Design review of the part built by this model. Coordinates are the model's own, in mm. A direction names the side the tool comes from. Coordinates: 2 decimals unless noted, no trailing zeros. Loops run counter-clockwise (first coordinate to the right, second up) from the corner with the lowest first, then second, coordinate; pieces in that order, holes last. Notation, with made-up numbers: (81, 71) -> (101, 71) arc R15 cw to (101, 91) -> close; hole circle Ø7 at (15, -8.75). An arc over 180 degrees is marked (long way). Use CSV: the item, a comma, the result in double quotes.
```python
from build123d import *

# Parameters (mm, degrees)
SKETCH2_W                                           = 240
SKETCH2_H                                           = 140
EXTRUDE1_DEPTH                                      = 12
CBORE_FOR_M4_HEX_SOCKET_HEAD_CAP_SCREW1_D           = 4.5
CBORE_FOR_M4_HEX_SOCKET_HEAD_CAP_SCREW1_CBORE_D     = 8
CBORE_FOR_M4_HEX_SOCKET_HEAD_CAP_SCREW1_CBORE_DEPTH = 4.4
CBORE_FOR_M6_HEX_SOCKET_HEAD_CAP_SCREW1_D           = 6.6
CBORE_FOR_M6_HEX_SOCKET_HEAD_CAP_SCREW1_CBORE_D     = 11
CBORE_FOR_M6_HEX_SOCKET_HEAD_CAP_SCREW1_CBORE_DEPTH = 6.4
CBORE_FOR_M6_HEX_SOCKET_HEAD_CAP_SCR_2_COUNT        = 2
CBORE_FOR_M6_HEX_SOCKET_HEAD_CAP_SCR_2_PITCH        = 35


with BuildPart() as part:
    # Sketch2 → Extrude1 (new body)
    with BuildSketch(Plane(origin=(0, 0, 0), x_dir=(1, 0, 0), z_dir=(0, 1, 0))):
        Rectangle(SKETCH2_W, SKETCH2_H)
    extrude(amount=EXTRUDE1_DEPTH)

    # CBORE for M4 Hex Socket Head Cap Screw1 (through all)
    with Locations(Plane(origin=(0, 12, 0), x_dir=(1, 0, 0), z_dir=(0, 1, 0))):
        with Locations((-95.5, 49), (-69.5, 49), (-69.5, 23), (-95.5, 23), (-95.5, -23), (-69.5, -23), (-69.5, -49), (-95.5, -49), (69.5, 49), (95.5, 49), (95.5, 23), (69.5, 23), (69.5, -23), (95.5, -23), (95.5, -49), (69.5, -49)):
            CounterBoreHole(CBORE_FOR_M4_HEX_SOCKET_HEAD_CAP_SCREW1_D / 2, CBORE_FOR_M4_HEX_SOCKET_HEAD_CAP_SCREW1_CBORE_D / 2, CBORE_FOR_M4_HEX_SOCKET_HEAD_CAP_SCREW1_CBORE_DEPTH)

    # CBORE for M6 Hex Socket Head Cap Screw1 (through all)
    with Locations(Plane(origin=(0, 0, 0), x_dir=(-1, 0, 0), z_dir=(0, -1, 0))):
        with Locations((110, -60), (110, 0), (110, 60), (55, 60), (55, 0), (55, -60), (-55, -60), (-55, 0), (-55, 60), (-110, 60), (-110, 0), (-110, -60)):
            CounterBoreHole(CBORE_FOR_M6_HEX_SOCKET_HEAD_CAP_SCREW1_D / 2, CBORE_FOR_M6_HEX_SOCKET_HEAD_CAP_SCREW1_CBORE_D / 2, CBORE_FOR_M6_HEX_SOCKET_HEAD_CAP_SCREW1_CBORE_DEPTH)

    # Sketch10 → CBORE for M6 Hex Socket Head Cap Screw2 (revolve, cut)
    with BuildSketch(Plane(origin=(17.5, 12, 12.8), x_dir=(0, 0, 1), z_dir=(1, 0, 0))):
        Polygon((0, 0), (0, 13.482840043), (3.3, 11.5), (3.3, 6.4), (5.5, 6.4), (5.5, 0.025), (5.525, 0), align=None)
    cbore_for_m6_hex_socket_head_cap_screw2 = revolve(axis=Axis((17.5, 18.35, 12.8), (0, -1, 0)), mode=Mode.SUBTRACT)

    # CBORE for M6 Hex Socket Head Cap Scr 2: CBORE for M6 Hex Socket Head Cap Screw2 ×2
    with Locations(*[(-i * CBORE_FOR_M6_HEX_SOCKET_HEAD_CAP_SCR_2_PITCH, 0, 0) for i in range(1, CBORE_FOR_M6_HEX_SOCKET_HEAD_CAP_SCR_2_COUNT)]):
        add(cbore_for_m6_hex_socket_head_cap_screw2, mode=Mode.SUBTRACT)


solid = part.part
```
Item 1: Add section B-B (y = 2.5). State how many separate pieces and enclosed holes the cut face has, then the cut area to 3 significant figures.
Checked values:
separate pieces,"1"
enclosed holes,"30"
area,"32,100 mm^2"
Item 2: Add section A-A (x = -110). Give the boundary of the cut face in (y, z).
Checked values:
outline,"(0, -70) -> (12, -70) -> (12, -63.3) -> (6.4, -63.3) -> (6.4, -65.5) -> (0, -65.5) -> close; (0, -54.5) -> (6.4, -54.5) -> (6.4, -56.7) -> (12, -56.7) -> (12, -3.3) -> (6.4, -3.3) -> (6.4, -5.5) -> (0, -5.5) -> close; (0, 5.5) -> (6.4, 5.5) -> (6.4, 3.3) -> (12, 3.3) -> (12, 56.7) -> (6.4, 56.7) -> (6.4, 54.5) -> (0, 54.5) -> close; (0, 65.5) -> (6.4, 65.5) -> (6.4, 63.3) -> (12, 63.3) -> (12, 70) -> (0, 70) -> close"
Item 3: To check wall thickness, follow line 1 along X through (y, z) = (10.55, 23); line 2 along X through (y, z) = (1.75, 0.5); line 3 along Z through (x, y) = (-55, 1.5). State the ranges of each line that lie inside material, in increasing order.
Checked values:
line 1,"-120 to -99.5, -91.5 to -73.5, -65.5 to 65.5, 73.5 to 91.5, 99.5 to 120"
line 2,"-120 to -115.48, -104.52 to -60.48, -49.52 to 49.52, 60.48 to 104.52, 115.48 to 120"
line 3,"-70 to -65.5, -54.5 to -5.5, 5.5 to 54.5, 65.5 to 70"
Item 4: Machinability: for faces 1 (the face through (-112.43, 9.24, -62.23)), 2 (the face through (106, 6.4, 0)), 3 (the face through (-94, 7.6, -21)), which of the approach directions +Z, -Z, +X, -X, +Y, -Y give a long, thin tool a straight path to every point of the face, cutting with its end or side? Answer none if there is none.
Checked values:
face 1,"+Y, -Y"
face 2,"-Y"
face 3,"+Y"
Item 5: Draft analysis for pull direction X (two halves, no side actions). For faces 4 (the face through (-120, 6, 1)), 5 (the face through (-49.505, 3.155, 59.758)), 6 (the face through (73.315, 9.831, 21.799)), state which applies: pulls with the +X half, pulls with the -X half, needs draft (parallel to the pull), parting line crosses it, or undercut.
Checked values:
face 4,"pulls with the -X half"
face 5,"undercut"
face 6,"undercut"
Item 6: Clearance check with flat-ended pins moving along their axes: pin 1 (8.5 mm diameter, centred on x = -55, z = 0, fed in from +Y); pin 2 (3.5 mm diameter, centred on x = -109.5, z = 1.5, fed in from -Y); pin 3 (10 mm diameter, centred on x = 17.5, z = 12.8, fed in from +Y); pin 4 (6 mm diameter, centred on x = -95.5, z = 49, fed in from +Y). State where each tip first meets the part, or that it passes through.
Checked values:
pin 1,"y = 12"
pin 2,"y = 6.4"
pin 3,"y = 5.6"
pin 4,"y = 7.6"
